Can you work these out from the model? Positions are in its coordinate system, mm. Round coordinates to 2 decimals unless told otherwise and drop trailing zeros. Write each loop counter-clockwise with the first axis right and the second up, starting at its lowest first coordinate (ties: lowest second). Pieces come first, ordered by that corner, then holes. Notation, with made-up numbers: M 24.5,87 L 40.5,87 A7 cw 40.5,93 Z; hole C 31.25,63.25 d8. An arc over 180 degrees is marked long. Answer in a Markdown table with one row per item. Add a question column.
(1) If I drill on probe 1 along X at (y, z) = (0.5, 42.5); probe 2 along Z at (x, y) = (81.5, 0.3); probe 3 along X at (y, z) = (-0.2, 68), over which ranges is the centre line in solid material (lowest first)?
(2) If we mould it in two halves opening along X, with no side actions, what happens to faces 1 (the face through (-2, -0.8, -18)), 2 (the face through (-4.88, -0.01, -1.08))? For each: released by +X, released by -X, zero draft, split by the parting line, or undercut.
(3) Suppose I cut it at B-B, the plane x = 66. Write out the boundary of the cut face in (y, z).
(4) I'm going to push flat-ended pins straight in: pin 1 (15 mm diameter, centred on x = 97, z = 0, fed in from +Y); pin 2 (0.5 mm diameter, centred on x = 37.5, y = 0.5, fed in from +Z). Where does each tip first touch, or does it pass through?
(5) Suppose I cut it at A-A, the plane y = -0.5. Count the separate pieces of the cut face and the enclosed holes in it, then the cut area to 3 significant figures.
from build123d import *

# Parameters (mm, degrees)
SKETCH_2_R          = 5
EXTRUDE_1_DEPTH     = 0.8
SKETCH_5_R          = 1.6
SKETCH_5_R_2        = 9.5
CUT_EXTRUDE_1_DEPTH = 2


with BuildPart() as part:
    # 草图2 → 凸台-拉伸1 (new, symmetric)
    with BuildSketch(Plane(origin=(0, 0, 0), x_dir=(1, 0, 0), z_dir=(0, 1, 0))):
        Polygon((-127.5, 75), (-127.5, -75), (-93.5, -75), (-93.5, -48), (-11, -48), (-11, -75), (11, -75), (11, -48), (93.5, -48), (93.5, -75), (127.5, -75), (127.5, 75), (93.5, 75), (93.5, 48), (11, 48), (11, 75), (-11, 75), (-11, 48), (-93.5, 48), (-93.5, 75), align=None)
        with Locations(Location((0, 0, 0), (0, 0, 270))):
            Circle(SKETCH_2_R, mode=Mode.SUBTRACT)
    extrude(amount=EXTRUDE_1_DEPTH, both=True)

    # 草图5 → 切除-拉伸1 (cut)
    with BuildSketch(Plane.XZ.offset(0.8)):
        with Locations(Location((-55.5, 0, 0), (0, 0, 270))):
            Circle(SKETCH_5_R)
        with Locations(Location((0, 56.5, 0), (0, 0, 270))):
            Circle(SKETCH_5_R)
        with Locations(Location((7, 70, 0), (0, 0, 270))):
            Circle(SKETCH_5_R)
        with Locations(Location((-7, 70, 0), (0, 0, 270))):
            Circle(SKETCH_5_R)
        with Locations(Location((99, 50, 0), (0, 0, 270))):
            Circle(SKETCH_5_R)
        with Locations(Location((-81.5, -42.5, 0), (0, 0, 270))):
            Circle(SKETCH_5_R)
        with Locations(Location((-50.5, -42.5, 0), (0, 0, 270))):
            Circle(SKETCH_5_R)
        with Locations(Location((-99, -50, 0), (0, 0, 270))):
            Circle(SKETCH_5_R)
        with Locations(Location((-97, 0, 0), (0, 0, 270))):
            Circle(SKETCH_5_R_2)
        with Locations(Location((-121.5, -7, 0), (0, 0, 270))):
            Circle(SKETCH_5_R)
        with Locations(Location((55.5, 0, 0), (0, 0, 90))):
            Circle(SKETCH_5_R)
        with Locations(Location((81.5, -42.5, 0), (0, 0, 90))):
            Circle(SKETCH_5_R)
        with Locations(Location((50.5, -42.5, 0), (0, 0, 90))):
            Circle(SKETCH_5_R)
        with Locations(Location((99, -50, 0), (0, 0, 90))):
            Circle(SKETCH_5_R)
        with Locations(Location((121.5, -7, 0), (0, 0, 90))):
            Circle(SKETCH_5_R)
        with Locations(Location((97, 0, 0), (0, 0, 270))):
            Circle(SKETCH_5_R_2)
        with Locations(Location((7, -70, 0), (0, 0, 90))):
            Circle(SKETCH_5_R)
        with Locations(Location((-7, -70, 0), (0, 0, 90))):
            Circle(SKETCH_5_R)
        with Locations(Location((0, -56.5, 0), (0, 0, 90))):
            Circle(SKETCH_5_R)
        with Locations(Location((50.5, 42.5, 0), (0, 0, 270))):
            Circle(SKETCH_5_R)
        with Locations(Location((81.5, 42.5, 0), (0, 0, 270))):
            Circle(SKETCH_5_R)
        with Locations(Location((121.5, 7, 0), (0, 0, 270))):
            Circle(SKETCH_5_R)
        with Locations(Location((-50.5, 42.5, 0), (0, 0, 90))):
            Circle(SKETCH_5_R)
        with Locations(Location((-121.5, 7, 0), (0, 0, 90))):
            Circle(SKETCH_5_R)
        with Locations(Location((-81.5, 42.5, 0), (0, 0, 90))):
            Circle(SKETCH_5_R)
        with Locations(Location((-99, 50, 0), (0, 0, 90))):
            Circle(SKETCH_5_R)
        with Locations(Location((-79.5, 19, 0), (0, 0, 270))):
            Circle(SKETCH_5_R)
        with Locations(Location((-41.5, 19, 0), (0, 0, 270))):
            Circle(SKETCH_5_R)
        with Locations(Location((-41.5, -19, 0), (0, 0, 90))):
            Circle(SKETCH_5_R)
        with Locations(Location((-79.5, -19, 0), (0, 0, 270))):
            Circle(SKETCH_5_R)
        with Locations(Location((41.5, 19, 0), (0, 0, 90))):
            Circle(SKETCH_5_R)
        with Locations(Location((79.5, 19, 0), (0, 0, 90))):
            Circle(SKETCH_5_R)
        with Locations(Location((41.5, -19, 0), (0, 0, 270))):
            Circle(SKETCH_5_R)
        with Locations(Location((79.5, -19, 0), (0, 0, 270))):
            Circle(SKETCH_5_R)
    extrude(amount=-CUT_EXTRUDE_1_DEPTH, mode=Mode.SUBTRACT)


solid = part.part
Calculated:
| question | item | result |
|---|---|---|
| 1 | probe 1 | -127.5 to -83.1, -79.9 to -52.1, -48.9 to 48.9, 52.1 to 79.9, 83.1 to 127.5 |
| 1 | probe 2 | -48 to -44.1, -40.9 to 40.9, 44.1 to 48 |
| 1 | probe 3 | -127.5 to -93.5, -11 to 11, 93.5 to 127.5 |
| 2 | face 1 | zero draft |
| 2 | face 2 | undercut |
| 3 | outline | M -0.8,-48 L 0.8,-48 L 0.8,48 L -0.8,48 Z |
| 4 | pin 1 | through |
| 4 | pin 2 | z = 48 |
| 5 | separate pieces | 1 |
| 5 | enclosed holes | 35 |
| 5 | area | 28,400 mm² |
